Part model, mm, in its own coordinate system. A direction names the side the tool comes from. Give positions to 0.01 mm unless a question says otherwise; leave off trailing zeros. Order: outer loops, then holes, each group sorted by start corner. A loop starts at its lowest first (then second) coordinate and runs counter-clockwise, first axis right, second up. Notation, with made-up numbers: (71.5, -16.5) - (129.5, -16.5) arc R17 cw to (129.5, -8.5) - close; hole circle Ø6 at (-21.75, -27). An arc over 180 degrees is marked (long way). One line per item, written item: value.
```python
from build123d import *

# Parameters (mm, degrees)
SKETCH1_W           = 60
SKETCH1_H           = 60
BOSS_EXTRUDE1_DEPTH = 18.87
FILLET1_R           = 10
SKETCH3_W           = 12
SKETCH3_H           = 25
CUT_EXTRUDE1_DEPTH  = 47.433575137
SKETCH5_R           = 1
CUT_EXTRUDE2_DEPTH  = 47.433575137
SKETCH8_R           = 1
CUT_EXTRUDE3_DEPTH  = 47.433575137


with BuildPart() as part:
    # Sketch1 → Boss-Extrude1 (new body)
    with BuildSketch(Plane(origin=(0, 0, 0), x_dir=(1, 0, 0), z_dir=(0, 1, 0))):
        Rectangle(SKETCH1_W, SKETCH1_H)
    extrude(amount=BOSS_EXTRUDE1_DEPTH)

    # Fillet1
    fillet1_edges = [part.edges().sort_by_distance(p)[0] for p in [
        (-30, 9.435, 30),
        (30, 9.435, 30),
        (30, 9.435, -30),
        (-30, 9.435, -30),
    ]]
    fillet(fillet1_edges, radius=FILLET1_R)

    # Sketch3 → Cut-Extrude1 (cut, through all)
    with BuildSketch(Plane(origin=(0, 0, 0), x_dir=(-1, 0, 0), z_dir=(0, -1, 0))):
        Rectangle(SKETCH3_W, SKETCH3_H)
    extrude(amount=-CUT_EXTRUDE1_DEPTH, mode=Mode.SUBTRACT)

    # Sketch5 → Cut-Extrude2 (cut, through all)
    with BuildSketch(Plane(origin=(0, 18.87, 0), x_dir=(1, 0, 0), z_dir=(0, 1, 0))):
        with Locations(Location((0, 13.7, 0), (0, 0, 270))):
            Circle(SKETCH5_R)
    extrude(amount=-CUT_EXTRUDE2_DEPTH, mode=Mode.SUBTRACT)

    # Sketch8 → Cut-Extrude3 (cut, through all)
    with BuildSketch(Plane(origin=(0, 18.87, 0), x_dir=(1, 0, 0), z_dir=(0, 1, 0))):
        with Locations(Location((0, -13.7, 0), (0, 0, 270))):
            Circle(SKETCH8_R)
    extrude(amount=-CUT_EXTRUDE3_DEPTH, mode=Mode.SUBTRACT)


solid = part.part
```
1) Which spindle directions (+Z, -Z, +X, -X, +Y, -Y) get a long thin tool onto all of the face, cutting with end or side? Do faces 1 (the flat face through (6.2, 18.87, -0.4)), 2 (the flat face through (6, 9, 0)). Say none if no direction does.
Outcome:
face 1: +Z, -Z, +X, -X, +Y
face 2: +Y, -Y
2) Cut at B-B, the plane z = -13.7. Give the cut face in (x, y), then the cut area to 3 significant figures.
Outcome:
outline: (-30, 0) - (-1, 0) - (-1, 18.87) - (-30, 18.87) - close; (1, 0) - (30, 0) - (30, 18.87) - (1, 18.87) - close
area: 1,090 mm^2
3) Cut at A-A, the plane x = 0. Give the cut face in (y, z).
Outcome:
outline: (0, -30) - (18.87, -30) - (18.87, -14.7) - (0, -14.7) - close; (0, -12.7) - (18.87, -12.7) - (18.87, -12.5) - (0, -12.5) - close; (0, 12.5) - (18.87, 12.5) - (18.87, 12.7) - (0, 12.7) - close; (0, 14.7) - (18.87, 14.7) - (18.87, 30) - (0, 30) - close
4) Mould opens along Z. For faces 3 (the flat face through (6.2, 0, -0.4)), 4 (the cylindrical face through (-27.15, 9.57, 26.99)), 5 (the flat face through (0, 9, -12.5)) say: released by +Z, released by -Z, zero draft, split by the parting line, or undercut.
Outcome:
face 3: zero draft
face 4: released by +Z
face 5: undercut
5) Drill centre lines: line 1 along X through (y, z) = (10.5, 13.7); line 2 along X through (y, z) = (6.5, -0.5); line 3 along Z through (x, y) = (27, 14.5). Where is each one in solid material? Low to high. Write a range as from..to.
Outcome:
line 1: x = -30..-1, 1..30
line 2: x = -30..-6, 6..30
line 3: z = -27.14..27.14
6) Cut at D-D, the plane z = 7. Give the cut face in (x, y), then the cut area to 3 significant figures.
Outcome:
outline: (-30, 0) - (-6, 0) - (-6, 18.87) - (-30, 18.87) - close; (6, 0) - (30, 0) - (30, 18.87) - (6, 18.87) - close
area: 906 mm^2
7) Cut at C-C, the plane y = 16. Give the cut face in (x, z).
Outcome:
outline: (-30, -20) arc R10 ccw to (-20, -30) - (20, -30) arc R10 ccw to (30, -20) - (30, 20) arc R10 ccw to (20, 30) - (-20, 30) arc R10 ccw to (-30, 20) - close; hole (-6, -12.5) - (6, -12.5) - (6, 12.5) - (-6, 12.5) - close; hole circle Ø2 at (0, -13.7); hole circle Ø2 at (0, 13.7)
